Model file for the job. Use its own axes, mm. A direction names the side the tool comes from. Coordinates: 2 decimals unless noted, no trailing zeros. Loops run counter-clockwise (first coordinate to the right, second up) from the corner with the lowest first, then second, coordinate; pieces in that order, holes last. Notation, with made-up numbers: M 69,-10 L 95,-10 A20 ccw 95,26 Z; hole C 44,52 d2. An arc over 180 degrees is marked long. Write item = value, one per line. Start each with the question number.
from build123d import *

# Parameters (mm, degrees)
SKETCH1_W           = 40
SKETCH1_H           = 40
SKETCH1_W_2         = 25.5
SKETCH1_H_2         = 25.5
BOSS_EXTRUDE1_DEPTH = 6
SKETCH5_R           = 1.7
CUT_EXTRUDE1_DEPTH  = 29.91366459
FILLET1_R           = 1


with BuildPart() as part:
    # Sketch1 → Boss-Extrude1 (new body)
    with BuildSketch(Plane(origin=(0, 0, 0), x_dir=(1, 0, 0), z_dir=(0, 1, 0))):
        Rectangle(SKETCH1_W, SKETCH1_H)
        Rectangle(SKETCH1_W_2, SKETCH1_H_2, mode=Mode.SUBTRACT)
    extrude(amount=BOSS_EXTRUDE1_DEPTH)

    # Sketch5 → Cut-Extrude1 (cut, through all)
    with BuildSketch(Plane.XZ.offset(-6)):
        with Locations(Location((-15, 15, 0), (0, 0, 270))):
            Circle(SKETCH5_R)
        with Locations(Location((-15, -15, 0), (0, 0, 270))):
            Circle(SKETCH5_R)
        with Locations(Location((15, -15, 0), (0, 0, 270))):
            Circle(SKETCH5_R)
        with Locations(Location((15, 15, 0), (0, 0, 270))):
            Circle(SKETCH5_R)
    extrude(amount=CUT_EXTRUDE1_DEPTH, mode=Mode.SUBTRACT)

    # Fillet1
    fillet1_edges = [part.edges().sort_by_distance(p)[0] for p in [
        (20, 3, 20),
        (-20, 3, 20),
        (-20, 3, -20),
        (20, 3, -20),
    ]]
    fillet(fillet1_edges, radius=FILLET1_R)


solid = part.part
Item 1: Cut at D-D (y = 4.2). Give the cut face in (x, z).
Item 2: Cut at C-C (z = -15). Give the cut face in (x, y).
Item 3: Pull direction X, two halves, no side cores. Call faces 1 (the flat face through (0, 6, -14)), 2 (the cylindrical face through (-19.715, 3.042, -19.699)), 3 (the cylindrical face through (19.699, 3.042, -19.715)), 4 (the cylindrical face through (-15.65, 3.04, -16.57)): +X half, -X half, draft (parallel to the pull), parting line (faces both ways), or undercut.
Item 4: Cut at B-B (z = -5.5). Give the cut face in (x, y).
Item 5: Cut at A-A (x = 8). Give the cut face in (y, z).
Item 6: Probe L1, parallel to Z at x = -15, y = 4.8; L2, parallel to X at y = 3.4, z = -8.5. List the from-to ranges inside material, lowest first.
Item 7: 3-axis set-ups, long thin cutter, end or side, ignore diameter. For faces 5 (the flat face through (0, 0, -14)), 6 (the flat face through (-12.75, 3, 0)): which of +Z, -Z, +X, -X, +Y, -Y reach the whole face in a straight line?
Reported:
q1.outline = M -20,-19 A1 ccw -19,-20 L 19,-20 A1 ccw 20,-19 L 20,19 A1 ccw 19,20 L -19,20 A1 ccw -20,19 Z; hole C -15,-15 d3.4; hole C -15,15 d3.4; hole M -12.75,-12.75 L 12.75,-12.75 L 12.75,12.75 L -12.75,12.75 Z; hole C 15,-15 d3.4; hole C 15,15 d3.4
q2.outline = M -20,0 L -16.7,0 L -16.7,6 L -20,6 Z; M -13.3,0 L 13.3,0 L 13.3,6 L -13.3,6 Z; M 16.7,0 L 20,0 L 20,6 L 16.7,6 Z
q3.face_1 = draft
q3.face_2 = -X half
q3.face_3 = +X half
q3.face_4 = undercut
q4.outline = M -20,0 L -12.75,0 L -12.75,6 L -20,6 Z; M 12.75,0 L 20,0 L 20,6 L 12.75,6 Z
q5.outline = M 0,-20 L 6,-20 L 6,-12.75 L 0,-12.75 Z; M 0,12.75 L 6,12.75 L 6,20 L 0,20 Z
q6.L1 = -20 to -16.7, -13.3 to 13.3, 16.7 to 20
q6.L2 = -20 to -12.75, 12.75 to 20
q7.face_5 = +Z, -Z, +X, -X, -Y
q7.face_6 = +Y, -Y
